from build123d import *

# Parameters (mm, degrees)
SKETCH1_W           = 190
SKETCH1_H           = 90
SKETCH1_R           = 1.5
SKETCH1_W_2         = 150
SKETCH1_H_2         = 50
BOSS_EXTRUDE1_DEPTH = 5
FILLET1_R           = 2
CUT_EXTRUDE1_DEPTH  = 106.237825899
SKETCH3_W           = 10
SKETCH3_H           = 10
BOSS_EXTRUDE2_DEPTH = 5


with BuildPart() as part:
    # Sketch1 → Boss-Extrude1 (new body)
    with BuildSketch(Plane(origin=(0, 0, 0), x_dir=(1, 0, 0), z_dir=(0, 1, 0))):
        Rectangle(SKETCH1_W, SKETCH1_H)
        with Locations(Location((-90, 40, 0), (0, 0, 270))):
            Circle(SKETCH1_R, mode=Mode.SUBTRACT)
        with Locations(Location((-90, -40, 0), (0, 0, 270))):
            Circle(SKETCH1_R, mode=Mode.SUBTRACT)
        with Locations(Location((90, 40, 0), (0, 0, 270))):
            Circle(SKETCH1_R, mode=Mode.SUBTRACT)
        with Locations(Location((90, -40, 0), (0, 0, 270))):
            Circle(SKETCH1_R, mode=Mode.SUBTRACT)
        Rectangle(SKETCH1_W_2, SKETCH1_H_2, mode=Mode.SUBTRACT)
    extrude(amount=BOSS_EXTRUDE1_DEPTH)

    # Fillet1
    fillet1_edges = [part.edges().sort_by_distance(p)[0] for p in [
        (-75, 2.5, -25),
        (-75, 2.5, 25),
        (75, 2.5, 25),
        (75, 2.5, -25),
    ]]
    fillet(fillet1_edges, radius=FILLET1_R)

    # Sketch2 → Cut-Extrude1 (cut, through all)
    with BuildSketch(Plane(origin=(0, 5, 0), x_dir=(1, 0, 0), z_dir=(0, 1, 0))):
        Polygon((95, -23.5), (90, -23.5), (90, -22.25), (87, -22.25), (87, -23.5), (84, -23.5), (84, -26.5), (87, -26.5), (87, -27.75), (90, -27.75), (90, -26.5), (95, -26.5), align=None)
        Polygon((95, 26.5), (95, 23.5), (90, 23.5), (90, 22.25), (87, 22.25), (87, 23.5), (84, 23.5), (84, 26.5), (87, 26.5), (87, 27.75), (90, 27.75), (90, 26.5), align=None)
        Polygon((-95, 23.5), (-90, 23.5), (-90, 22.25), (-87, 22.25), (-87, 23.5), (-84, 23.5), (-84, 26.5), (-87, 26.5), (-87, 27.75), (-90, 27.75), (-90, 26.5), (-95, 26.5), align=None)
        Polygon((-95, -26.5), (-95, -23.5), (-90, -23.5), (-90, -22.25), (-87, -22.25), (-87, -23.5), (-84, -23.5), (-84, -26.5), (-87, -26.5), (-87, -27.75), (-90, -27.75), (-90, -26.5), align=None)
    extrude(amount=-CUT_EXTRUDE1_DEPTH, mode=Mode.SUBTRACT)

    # Sketch3 → Boss-Extrude2 (add)
    with BuildSketch(Plane(origin=(0, 5, 0), x_dir=(1, 0, 0), z_dir=(0, 1, 0))):
        with Locations((100, 40)):
            Rectangle(SKETCH3_W, SKETCH3_H)
        with Locations((100, 0)):
            Rectangle(SKETCH3_W, SKETCH3_H)
        with Locations((100, -40)):
            Rectangle(SKETCH3_W, SKETCH3_H)
        with Locations((-100, -40)):
            Rectangle(SKETCH3_W, SKETCH3_H)
        with Locations((-100, 0)):
            Rectangle(SKETCH3_W, SKETCH3_H)
        with Locations((-100, 40)):
            Rectangle(SKETCH3_W, SKETCH3_H)
    extrude(amount=-BOSS_EXTRUDE2_DEPTH)


solid = part.part
Here's how the part is built. I have some questions about the finished solid (model axes, mm). A direction names the side the tool comes from. Give positions to 0.01 mm unless a question says otherwise; leave off trailing zeros. Order: outer loops, then holes, each group sorted by start corner. A loop starts at its lowest first (then second) coordinate and runs counter-clockwise, first axis right, second up. Notation, with made-up numbers: (47, -35.5) -> (83, -35.5) arc R19 ccw to (83, -24.5) -> close; hole circle Ø7 at (88, 29). An arc over 180 degrees is marked (long way). One line per item, written item: value. Start each with the question number.
1. Imagine slicing it at A-A, the plane x = 41. List the corners of the cut face in (y, z) for me.
2. We'd pull the mould along Z, two halves only. Please class faces 1 (the face through (-105, 3, -40)), 2 (the face through (-92, 3, 26.5)), 3 (the face through (95, 2, 31)), 4 (the face through (-1, 2, 45)): released by +Z, released by -Z, zero draft, split by the parting line, or undercut.
3. For faces 5 (the face through (-95, 2, 14)), 6 (the face through (-105, 3, 40)), 7 (the face through (93, 3, 23.5)), 8 (the face through (75, 2, 0)), which set-ups out of +Z, -Z, +X, -X, +Y, -Y let a thin tool reach every point of the face, with its end or its side?
4. Will these pins go through, and if not, where does the flat tip stop? pin 1 Ø1 at (y, z) = (3, -26.5) entering from +X; pin 2 Ø2.5 at (y, z) = (2.5, -8.5) entering from -X.
5. I need wall thicknesses on probe 1 along X at (y, z) = (2.75, -40); probe 2 along Z at (x, y) = (-93, 1.05); probe 3 along X at (y, z) = (3.15, 27). Which ranges of each line are inside material? Lowest first, please. Write a range as from..to.
6. Imagine slicing it at C-C, the plane y = 1.8. Count the separate pieces of the cut face and the enclosed holes in it, plus the area to 3 significant figures.
7. Imagine slicing it at B-B, the plane z = -10. List the corners of the cut face in (x, y) for me, plus the area to 3 significant figures.
Values follow:
1. outline: (0, -45) -> (5, -45) -> (5, -25) -> (0, -25) -> close; (0, 25) -> (5, 25) -> (5, 45) -> (0, 45) -> close
2. face 1: zero draft
2. face 2: undercut
2. face 3: undercut
2. face 4: released by +Z
3. face 5: -X, +Y, -Y
3. face 6: +Z, -Z, -X, +Y, -Y
3. face 7: +X, +Y, -Y
3. face 8: +Y, -Y
4. pin 1: stops at x = 95
4. pin 2: stops at x = -95
5. probe 1: x = -105..-91.5, -88.5..88.5, 91.5..105
5. probe 2: z = -45..-26.5, -23.5..23.5, 26.5..45
5. probe 3: x = -95..-90, -87..87, 90..95
6. separate pieces: 1
6. enclosed holes: 5
6. area: 10,000 mm2
7. outline: (-95, 0) -> (-75, 0) -> (-75, 5) -> (-95, 5) -> close; (75, 0) -> (95, 0) -> (95, 5) -> (75, 5) -> close
7. area: 200 mm2
